The drawing under review shows one solid part. Ordinate dimensions are in mm from its lowest x, y, z. Coordinates: 2 decimals unless noted, no trailing zeros. Loops run counter-clockwise (first coordinate to the right, second up) from the corner with the lowest first, then second, coordinate; pieces in that order, holes last. Notation, with made-up numbers: M 19,-22.5 L 75,-22.5 A9 cw 75,-16.5 Z; hole C 76.5,-21 d4. An arc over 180 degrees is marked long. Return JSON: item names as keys, results as strings.
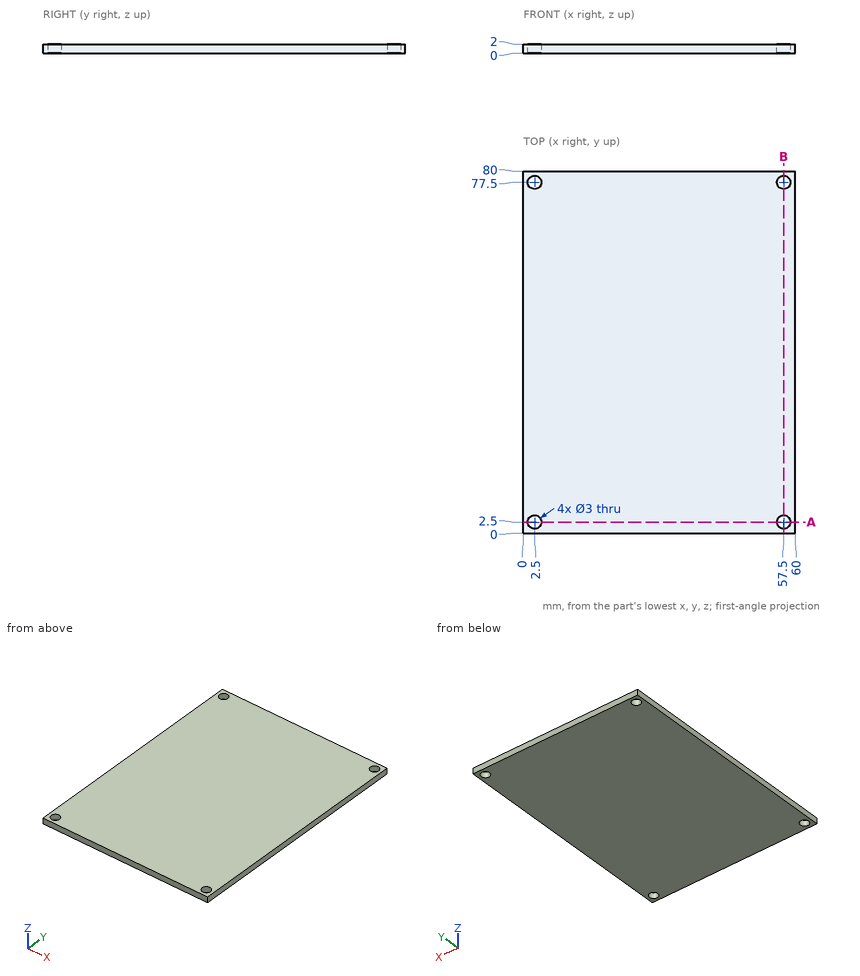
1. To check wall thickness, follow line 1 (Y direction, x = 2.5, z = 1); line 2 (X direction, y = 77.5, z = 0.9); line 3 (Y direction, x = 3, z = 0.75). State the ranges of each line that lie inside material, in increasing order.
Check values:
{"line 1": "0 to 1, 4 to 76, 79 to 80", "line 2": "0 to 1, 4 to 56, 59 to 60", "line 3": "0 to 1.09, 3.91 to 76.09, 78.91 to 80"}
2. Add section A-A on y = 2.5. Give the boundary of the cut face in (x, z).
Check values:
{"outline": "M 0,0 L 1,0 L 1,2 L 0,2 Z; M 4,0 L 56,0 L 56,2 L 4,2 Z; M 59,0 L 60,0 L 60,2 L 59,2 Z"}
3. Add section B-B on x = 57.5. Give the boundary of the cut face in (y, z).
Check values:
{"outline": "M 0,0 L 1,0 L 1,2 L 0,2 Z; M 4,0 L 76,0 L 76,2 L 4,2 Z; M 79,0 L 80,0 L 80,2 L 79,2 Z"}
